The figure shows three views and two pictorial views of one solid part (mm, origin at its lowest corner). Answer the questions. Round coordinates to 2 decimals unless told otherwise and drop trailing zeros. Loops run counter-clockwise (first coordinate to the right, second up) from the corner with the lowest first, then second, coordinate; pieces in that order, holes last. Notation, with made-up numbers: (38, 46.5) -> (43, 46.5) arc R18 cw to (43, 77.5) -> close; hole circle Ø1 at (-39, -6.5). An arc over 180 degrees is marked (long way). Use a Markdown table: item, result. Add a question column.
Q1. Section D-D on x = 90 is taken. Give the vertices of the cut face in (y, z) (1 decimal).
Q2. Section A-A on x = 61 is taken. Give the vertices of the cut face in (y, z).
Q3. For a pull along Z with two mould halves and no side action, classify the marked faces 1 and 2 as released by +Z, released by -Z, zero draft, split by the parting line, or undercut.
Q4. Section B-B on y = 61 is taken. Give the vertices of the cut face in (x, z), then the cut area to 3 significant figures.
Q5. Consider line 1 (Y direction, x = 89, z = 1.65) (1 decimal); line 2 (Y direction, x = 32, z = 0.6) (1 decimal); line 3 (X direction, y = 81, z = 1). Determine where each line is inside the solid, lowest interval first.
Q6. Section C-C on y = 75.5 is taken. Give the vertices of the cut face in (x, z) (1 decimal).
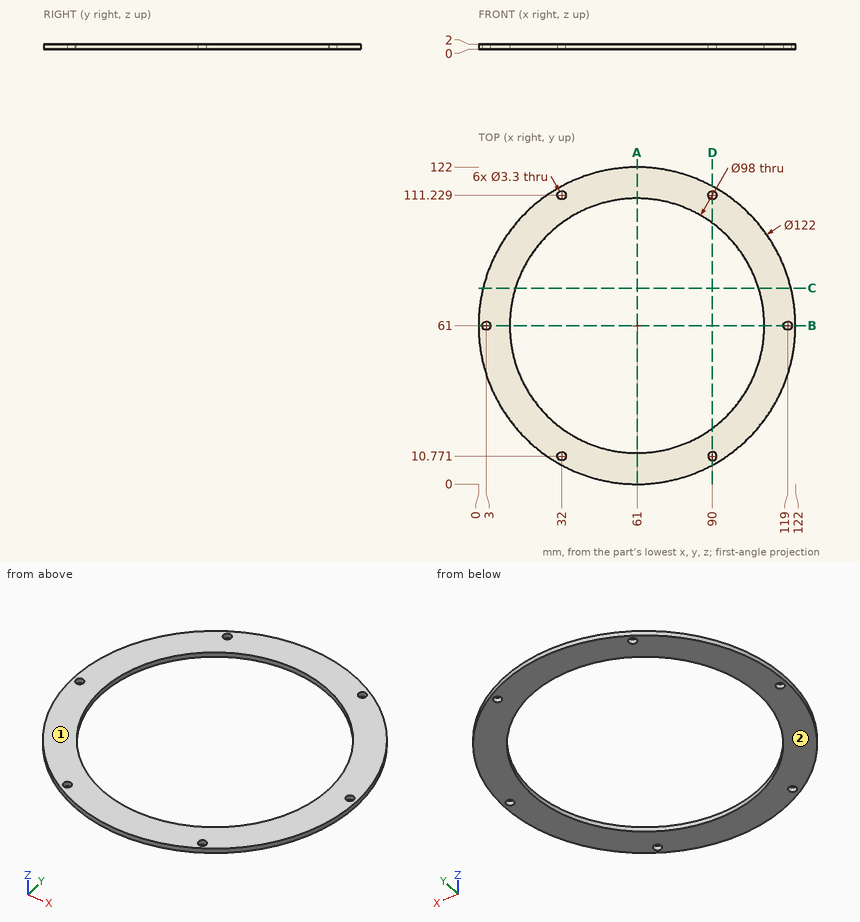
Checked values:
| question | item | result |
|---|---|---|
| 1 | outline | (7.3, 0) -> (9.1, 0) -> (9.1, 2) -> (7.3, 2) -> close; (12.4, 0) -> (21.5, 0) -> (21.5, 2) -> (12.4, 2) -> close; (100.5, 0) -> (109.6, 0) -> (109.6, 2) -> (100.5, 2) -> close; (112.9, 0) -> (114.7, 0) -> (114.7, 2) -> (112.9, 2) -> close |
| 2 | outline | (0, 0) -> (12, 0) -> (12, 2) -> (0, 2) -> close; (110, 0) -> (122, 0) -> (122, 2) -> (110, 2) -> close |
| 3 | face 1 | released by +Z |
| 3 | face 2 | released by -Z |
| 4 | outline | (0, 0) -> (1.35, 0) -> (1.35, 2) -> (0, 2) -> close; (4.65, 0) -> (12, 0) -> (12, 2) -> (4.65, 2) -> close; (110, 0) -> (117.35, 0) -> (117.35, 2) -> (110, 2) -> close; (120.65, 0) -> (122, 0) -> (122, 2) -> (120.65, 2) -> close |
| 4 | area | 34.8 mm2 |
| 5 | line 1 | y = 6.8 to 9.5, 12.1 to 20.8, 101.2 to 109.9, 112.5 to 115.2 |
| 5 | line 2 | y = 7.3 to 9.1, 12.4 to 21.5, 100.5 to 109.6, 112.9 to 114.7 |
| 5 | line 3 | x = 3.37 to 16.27, 105.73 to 118.63 |
| 6 | outline | (1.7, 0) -> (14.2, 0) -> (14.2, 2) -> (1.7, 2) -> close; (107.8, 0) -> (120.3, 0) -> (120.3, 2) -> (107.8, 2) -> close |
